Verification items for the finished model (mm, model axes). A direction names the side the tool comes from. Coordinates: 2 decimals unless noted, no trailing zeros. Write each loop counter-clockwise with the first axis right and the second up, starting at its lowest first coordinate (ties: lowest second). Pieces come first, ordered by that corner, then holes. Notation, with made-up numbers: M 3.25,60.25 L 31.25,60.25 A23 ccw 31.25,72.25 Z; hole C -37.5,35.5 d8. An arc over 180 degrees is marked long. Answer in a Markdown table with one row per item.
from build123d import *

# Parameters (mm, degrees)
SKETCH1_W           = 42.3
SKETCH1_H           = 42.3
BOSS_EXTRUDE1_DEPTH = 60
SKETCH2_R           = 1.5
CUT_EXTRUDE1_DEPTH  = 4.5
SKETCH3_W           = 70.080041738
SKETCH3_H           = 62.101106944
SKETCH3_R           = 27
CUT_EXTRUDE2_DEPTH  = 68.04211363
SKETCH4_R           = 11
BOSS_EXTRUDE2_DEPTH = 2
SKETCH5_R           = 2.5
BOSS_EXTRUDE3_DEPTH = 24
CHAMFER1_SIZE       = 0.5


with BuildPart() as part:
    # Sketch1 → Boss-Extrude1 (new body)
    with BuildSketch(Plane.XY):
        Rectangle(SKETCH1_W, SKETCH1_H)
    extrude(amount=BOSS_EXTRUDE1_DEPTH)

    # Sketch2 → Cut-Extrude1 (cut)
    with BuildSketch(Plane.XY.offset(60)):
        with Locations((-15.5, 15.5)):
            Circle(SKETCH2_R)
        with Locations((-15.5, -15.5)):
            Circle(SKETCH2_R)
        with Locations((15.5, -15.5)):
            Circle(SKETCH2_R)
        with Locations((15.5, 15.5)):
            Circle(SKETCH2_R)
    extrude(amount=-CUT_EXTRUDE1_DEPTH, mode=Mode.SUBTRACT)

    # Sketch3 → Cut-Extrude2 (cut, through all)
    with BuildSketch(Plane.XY.offset(60)):
        Rectangle(SKETCH3_W, SKETCH3_H)
        Circle(SKETCH3_R, mode=Mode.SUBTRACT)
    extrude(amount=-CUT_EXTRUDE2_DEPTH, mode=Mode.SUBTRACT)

    # Sketch4 → Boss-Extrude2 (add)
    with BuildSketch(Plane.XY.offset(60)):
        Circle(SKETCH4_R)
    extrude(amount=BOSS_EXTRUDE2_DEPTH)

    # Sketch5 → Boss-Extrude3 (add)
    with BuildSketch(Plane.XY.offset(60)):
        Circle(SKETCH5_R)
    extrude(amount=BOSS_EXTRUDE3_DEPTH)

    # Chamfer1
    chamfer1_edges = [part.edges().sort_by_distance(p)[0] for p in [
        (-2.5, 0, 84),
    ]]
    chamfer(chamfer1_edges, length=CHAMFER1_SIZE)


solid = part.part
1) Sectioned sample at A-A (x = 0). Record the cut outline in (y, z), then the cut area to 3 significant figures.
Response values:
| item | result |
|---|---|
| outline | M -21.15,0 L 21.15,0 L 21.15,60 L 11,60 L 11,62 L 2.5,62 L 2.5,83.5 L 2,84 L -2,84 L -2.5,83.5 L -2.5,62 L -11,62 L -11,60 L -21.15,60 Z |
| area | 2,690 mm² |
2) Tool access check on faces 1 (the face through (21.15, 0, 30)), 2 (the face through (-17, -15.43, 57.78)). Record the directions out of +Z, -Z, +X, -X, +Y, -Y that give a thin tool (end or side, any length) a straight path to the whole face; none if there is none.
Response values:
| item | result |
|---|---|
| face 1 | +Z, -Z, +X, +Y, -Y |
| face 2 | +Z |
3) Sectioned sample at D-D (y = -15.5). Record the cut outline in (x, z).
Response values:
| item | result |
|---|---|
| outline | M -21.15,0 L 21.15,0 L 21.15,60 L 17,60 L 17,55.5 L 14,55.5 L 14,60 L -14,60 L -14,55.5 L -17,55.5 L -17,60 L -21.15,60 Z |
4) Release check for a two-part mould opening along Y. For faces 3 (the face through (-16, -15, 55.5)), 4 (the face through (-0.54, -2.44, 72.6)), 5 (the face through (19.122, 19.061, 30.42)) record: +Y half, -Y half, draft (parallel to the pull), parting line (faces both ways), or undercut.
Response values:
| item | result |
|---|---|
| face 3 | undercut |
| face 4 | parting line |
| face 5 | +Y half |
5) Sectioned sample at C-C (z = 24.5). Record the cut outline in (x, y), then the cut area to 3 significant figures.
Response values:
| item | result |
|---|---|
| outline | M -21.15,-16.78 A27 ccw -16.78,-21.15 L 16.78,-21.15 A27 ccw 21.15,-16.78 L 21.15,16.78 A27 ccw 16.78,21.15 L -16.78,21.15 A27 ccw -21.15,16.78 Z |
| area | 1,750 mm² |
6) Thickness scan on L1, parallel to Y at x = -15.5, z = 57.55; L2, parallel to X at y = -15, z = 56. Record the ranges inside material, lowest first. Write a range as [from, to].
Response values:
| item | result |
|---|---|
| L1 | y = [-21.15, -17], [-14, 14], [17, 21.15] |
| L2 | x = [-21.15, -16.91], [-14.09, 14.09], [16.91, 21.15] |
7) Sectioned sample at B-B (y = -8). Record the cut outline in (x, z), then the cut area to 3 significant figures.
Response values:
| item | result |
|---|---|
| outline | M -21.15,0 L 21.15,0 L 21.15,60 L 7.55,60 L 7.55,62 L -7.55,62 L -7.55,60 L -21.15,60 Z |
| area | 2,570 mm² |
8) Depth check by flat-ended pin: pin 1 (3.5 mm diameter, centred on x = 16, y = -16, fed in from +Z); pin 2 (1.8 mm diameter, centred on x = -15.5, y = -15.5, fed in from +Z); pin 3 (2 mm diameter, centred on x = 1.5, y = 5.5, fed in from +Z). Enter the tip coordinate at first touch or a pass-through.
Response values:
| item | result |
|---|---|
| pin 1 | stops at z = 60 |
| pin 2 | stops at z = 55.5 |
| pin 3 | stops at z = 62 |
